Source: CAD feature listing. Evaluate the final solid. Frame: model axes, mm. Face numbers are marked on the shaded views. A direction names the side the tool comes from. Coordinates: 2 decimals unless noted, no trailing zeros. Loops run counter-clockwise (first coordinate to the right, second up) from the corner with the lowest first, then second, coordinate; pieces in that order, holes last. Notation, with made-up numbers: M 43.25,-20 L 92.25,-20 A22 ccw 92.25,12 Z; hole C -9.75,-6 d1. An arc over 180 degrees is marked long. One line per question, with ' | ' between items. Start each with the question number.
1. Ray query, probe 1 along Z at (x, y) = (12.5, -13.5); probe 2 along X at (y, z) = (61.5, -0.25); probe 3 along Y at (x, z) = (0, 1.25). Return the intervals inside material, ascending.
2. Access query for the marked faces 4, 5, 6 and 7. Directions: +Z, -Z, +X, -X, +Y, -Y. A direction counts if a zero-diameter tool reaches every point of the face in a straight line with its end or side. Return the directions, or none.
3. Section query A-A, the plane y = 32.5. Output: boundary loops of the cut face in (x, z).
4. Pin query (flat end, axial travel): P1, Ø4, axis at y = 45.5, z = 1, coming from the +X side; P2, Ø1, axis at x = -14.5, y = 57.5, coming from the -Z side (3 decimals); P3, Ø3, axis at y = -1, z = 6.5, coming from the +X side; P4, Ø8.5, axis at x = 0, y = 57.94, coming from the +Z side. Return the tip coordinate at first contact, or that it passes through.
5. Mould query, pull axis Z, two halves, no side actions, for the marked faces 1, 2 and 3. Classes: pulls with the +Z half, pulls with the -Z half, needs draft (parallel to the pull), parting line crosses it, or undercut.
6. Section query B-B, the plane x = 0. State how many separate pieces and enclosed holes the cut face has, and give its area (3 significant figures).
```python
from build123d import *

# Parameters (mm, degrees)
BOSS_EXTRUDE1_DEPTH = 1.5875
SKETCH5_W           = 28.575
SKETCH5_H           = 13.335
BOSS_EXTRUDE2_DEPTH = 6.31825
SKETCH32_R          = 4.7625
BOSS_EXTRUDE9_DEPTH = 3.175
SKETCH6_R           = 3.96875
SKETCH6_R_2         = 2.921
BOSS_EXTRUDE3_DEPTH = 1.778
DOME1_FACE_RADIUS   = 2.921
DOME1_HEIGHT        = 1.016
DOME3_FACE_RADIUS   = 2.921
DOME3_HEIGHT        = 1.016
DOME4_FACE_RADIUS   = 3.96875
DOME4_HEIGHT        = 1.016
SKETCH8_R           = 4.191
SKETCH8_R_2         = 6.35
BOSS_EXTRUDE4_DEPTH = 1.778
DOME5_FACE_RADIUS   = 4.191
DOME5_HEIGHT        = 2.54
DOME6_FACE_RADIUS   = 4.191
DOME6_HEIGHT        = 2.54
DOME7_FACE_RADIUS   = 6.35
DOME7_HEIGHT        = 3.9624
SKETCH9_R           = 3.57505
BOSS_EXTRUDE5_DEPTH = 15.8115


with BuildPart() as part:
    # Sketch3 → Revolve1 (revolve)
    with BuildSketch(Plane(origin=(0, 0, 0), x_dir=(0, 0, -1), z_dir=(1, 0, 0)), mode=Mode.PRIVATE) as revolve1_sk:
        with BuildLine():
            Line((-5.55625, 25.4), (-5.55625, 0))
            Line((-5.55625, 0), (5.55625, 0))
            Line((5.55625, 0), (5.55625, 25.4))
            Line((5.55625, 25.4), (2.559789657, 25.4))
            Line((2.559789657, 25.4), (2.372188625, 23.255710388))
            ThreePointArc((2.372188625, 23.255710388), (0, 21.082), (-2.372188625, 23.255710388))
            Line((-2.372188625, 23.255710388), (-2.559789657, 25.4))
            Line((-2.559789657, 25.4), (-5.55625, 25.4))
        make_face()
    revolve(revolve1_sk.sketch.rotate(Axis((0, 0, 5.55625), (0, 0, -1)), 90), axis=Axis((0, 0, 5.55625), (0, 0, -1)))



with BuildPart() as body_2:
    # Sketch4 → Boss-Extrude1 (new body)
    with BuildSketch(Plane.XY.offset(6.31825)):
        with BuildLine():
            Line((14.2875, 47.625), (-14.2875, 47.625))
            Line((-14.2875, 47.625), (-25.919465871, 7.517076905))
            ThreePointArc((-25.919465871, 7.517076905), (0, -26.9875), (25.919465871, 7.517076905))
            Line((25.919465871, 7.517076905), (14.2875, 47.625))
        make_face()
    extrude(amount=BOSS_EXTRUDE1_DEPTH)

    # Sketch5 → Boss-Extrude2 (add)
    with BuildSketch(Plane(origin=(0, 0, 6.31825), x_dir=(-1, 0, 0), z_dir=(0, 0, -1))):
        with Locations((0, 40.9575)):
            Rectangle(SKETCH5_W, SKETCH5_H)
    extrude(amount=BOSS_EXTRUDE2_DEPTH)

    # Mirror1: body 2 across plane


with BuildPart() as body_2_1:
    add(body_2.part)
    add(body_2.part.mirror(Plane.XY))

    # Sketch32 → Boss-Extrude9 (add, symmetric)
    with BuildSketch(Plane.XY):
        with BuildLine():
            Line((14.2875, 63.5), (14.2875, 34.29))
            Line((14.2875, 34.29), (-14.2875, 34.29))
            Line((-14.2875, 34.29), (-14.2875, 63.5))
            ThreePointArc((-14.2875, 63.5), (0, 68.2625), (14.2875, 63.5))
        make_face()
        with Locations((0, 57.94375)):
            Circle(SKETCH32_R, mode=Mode.SUBTRACT)
    extrude(amount=BOSS_EXTRUDE9_DEPTH, both=True)

    # Sketch6 → Boss-Extrude3 (add)
    with BuildSketch(Plane.XY.offset(7.90575)):
        Circle(SKETCH6_R)
        with Locations((-8.5725, 40.9575)):
            Circle(SKETCH6_R_2)
        with Locations((8.5725, 40.9575)):
            Circle(SKETCH6_R_2)
    extrude(amount=BOSS_EXTRUDE3_DEPTH)

    # Dome1: a dome of height H over a round flat face of radius A is a cap of a sphere of radius (A * A + H * H) / (2 * H)
    dome1_r = (DOME1_FACE_RADIUS * DOME1_FACE_RADIUS + DOME1_HEIGHT * DOME1_HEIGHT) / (2 * DOME1_HEIGHT)
    dome1_base = Plane((-8.5725, 40.9575, 9.68375), z_dir=(0, 0, 1))
    with Locations(dome1_base.offset(DOME1_HEIGHT - dome1_r)):
        dome1_ball = Sphere(dome1_r, mode=Mode.PRIVATE)
    add(split(dome1_ball, bisect_by=dome1_base, keep=Keep.TOP, mode=Mode.PRIVATE))

    # Dome3: a dome of height H over a round flat face of radius A is a cap of a sphere of radius (A * A + H * H) / (2 * H)
    dome3_r = (DOME3_FACE_RADIUS * DOME3_FACE_RADIUS + DOME3_HEIGHT * DOME3_HEIGHT) / (2 * DOME3_HEIGHT)
    dome3_base = Plane((8.5725, 40.9575, 9.68375), z_dir=(0, 0, 1))
    with Locations(dome3_base.offset(DOME3_HEIGHT - dome3_r)):
        dome3_ball = Sphere(dome3_r, mode=Mode.PRIVATE)
    add(split(dome3_ball, bisect_by=dome3_base, keep=Keep.TOP, mode=Mode.PRIVATE))

    # Dome4: a dome of height H over a round flat face of radius A is a cap of a sphere of radius (A * A + H * H) / (2 * H)
    dome4_r = (DOME4_FACE_RADIUS * DOME4_FACE_RADIUS + DOME4_HEIGHT * DOME4_HEIGHT) / (2 * DOME4_HEIGHT)
    dome4_base = Plane((0, 0, 9.68375), z_dir=(0, 0, 1))
    with Locations(dome4_base.offset(DOME4_HEIGHT - dome4_r)):
        dome4_ball = Sphere(dome4_r, mode=Mode.PRIVATE)
    add(split(dome4_ball, bisect_by=dome4_base, keep=Keep.TOP, mode=Mode.PRIVATE))

    # Sketch8 → Boss-Extrude4 (add)
    with BuildSketch(Plane(origin=(0, 0, -7.90575), x_dir=(-1, 0, 0), z_dir=(0, 0, -1))):
        with Locations((-8.5725, 40.9575)):
            Circle(SKETCH8_R)
        with Locations((8.5725, 40.9575)):
            Circle(SKETCH8_R)
        Circle(SKETCH8_R_2)
    extrude(amount=BOSS_EXTRUDE4_DEPTH)

    # Dome5: a dome of height H over a round flat face of radius A is a cap of a sphere of radius (A * A + H * H) / (2 * H)
    dome5_r = (DOME5_FACE_RADIUS * DOME5_FACE_RADIUS + DOME5_HEIGHT * DOME5_HEIGHT) / (2 * DOME5_HEIGHT)
    dome5_base = Plane((8.5725, 40.9575, -9.68375), z_dir=(0, 0, -1))
    with Locations(dome5_base.offset(DOME5_HEIGHT - dome5_r)):
        dome5_ball = Sphere(dome5_r, mode=Mode.PRIVATE)
    add(split(dome5_ball, bisect_by=dome5_base, keep=Keep.TOP, mode=Mode.PRIVATE))

    # Dome6: a dome of height H over a round flat face of radius A is a cap of a sphere of radius (A * A + H * H) / (2 * H)
    dome6_r = (DOME6_FACE_RADIUS * DOME6_FACE_RADIUS + DOME6_HEIGHT * DOME6_HEIGHT) / (2 * DOME6_HEIGHT)
    dome6_base = Plane((-8.5725, 40.9575, -9.68375), z_dir=(0, 0, -1))
    with Locations(dome6_base.offset(DOME6_HEIGHT - dome6_r)):
        dome6_ball = Sphere(dome6_r, mode=Mode.PRIVATE)
    add(split(dome6_ball, bisect_by=dome6_base, keep=Keep.TOP, mode=Mode.PRIVATE))

    # Dome7: a dome of height H over a round flat face of radius A is a cap of a sphere of radius (A * A + H * H) / (2 * H)
    dome7_r = (DOME7_FACE_RADIUS * DOME7_FACE_RADIUS + DOME7_HEIGHT * DOME7_HEIGHT) / (2 * DOME7_HEIGHT)
    dome7_base = Plane((0, 0, -9.68375), z_dir=(0, 0, -1))
    with Locations(dome7_base.offset(DOME7_HEIGHT - dome7_r)):
        dome7_ball = Sphere(dome7_r, mode=Mode.PRIVATE)
    add(split(dome7_ball, bisect_by=dome7_base, keep=Keep.TOP, mode=Mode.PRIVATE))


with BuildPart() as part_1:
    add(part.part)

    add(body_2_1.part)  # Boss-Extrude5 merges body 2
    # Sketch9 → Boss-Extrude5 (add)
    with BuildSketch(Plane.XY.offset(7.90575)):
        Circle(SKETCH9_R)
    extrude(amount=-BOSS_EXTRUDE5_DEPTH)


solid = part_1.part
```
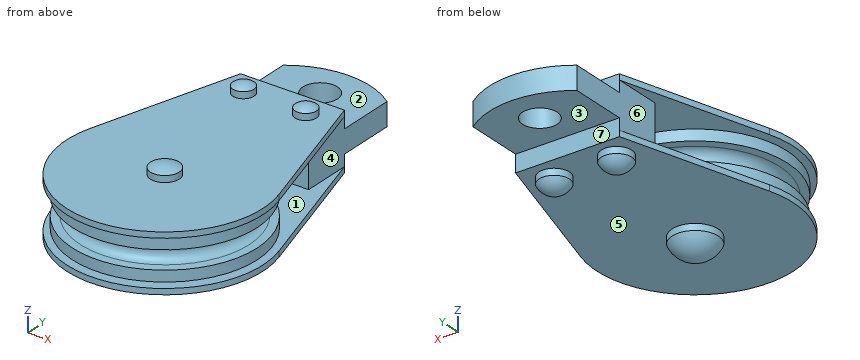
Taken from the geometry:
1) probe 1: -7.91 to -6.32, -5.56 to 5.56, 6.32 to 7.91 | probe 2: -14.29 to -3.17, 3.17 to 14.29 | probe 3: -21.44 to 21.44, 34.29 to 53.18, 62.71 to 68.26
2) face 4: +X, +Y | face 5: -Z | face 6: -X, +Y | face 7: -Z, +X, -X, +Y
3) outline: M -18.67,-7.91 L 18.67,-7.91 L 18.67,-6.32 L -18.67,-6.32 Z; M -18.67,6.32 L 18.67,6.32 L 18.67,7.91 L -18.67,7.91 Z
4) P1: x = 14.29 | P2: z = -3.175 | P3: x = 26.99 | P4: through
5) face 1: undercut | face 2: pulls with the +Z half | face 3: pulls with the -Z half
6) separate pieces: 2 | enclosed holes: 1 | area: 1,090 mm^2
